Study the drawing (mm; zero at the part's minimum x, y, z) and answer. A direction names the side the tool comes from. Give positions to 0.01 mm unless a question says otherwise; leave off trailing zeros. Write each loop counter-clockwise with the first axis right and the second up, starting at its lowest first coordinate (ties: lowest second). Pieces come first, ordered by that corner, then holes. Notation, with made-up numbers: M -25,-27 L 10,-27 A12 ccw 10,-11 Z; hole C 36,-28.75 d4. An arc over 180 degrees is marked long. Use a Markdown table: item, result. Add a question column.
Item 1: Given P1, Ø2, axis at x = 5, z = 6.5, coming from the +Y side (3 decimals); P2, Ø4, axis at y = 2, z = 3.5, coming from the +X side; P3, Ø4, axis at y = 1, z = 6, coming from the -X side, each flat-ended and moving along its own axis, determine where each tip first touches the part or whether it passes through.
Item 2: A cutting plane is placed at A-A on z = 10.75. Determine the outline of the cut face in (x, y), then the cut area to 3 significant figures.
Item 3: Consider probe 1 along Y at (x, z) = (4, 3.5); probe 2 along Z at (x, y) = (6, 4.75); probe 3 along X at (y, z) = (4.5, 13). Determine where each line is inside the solid, lowest interval first. Write a range as [from, to].
Item 4: For the marked faces 1 and 2, determine the directions among +Z, -Z, +X, -X, +Y, -Y from which every point of the face is accessible in a straight line to the end or side of a thin tool.
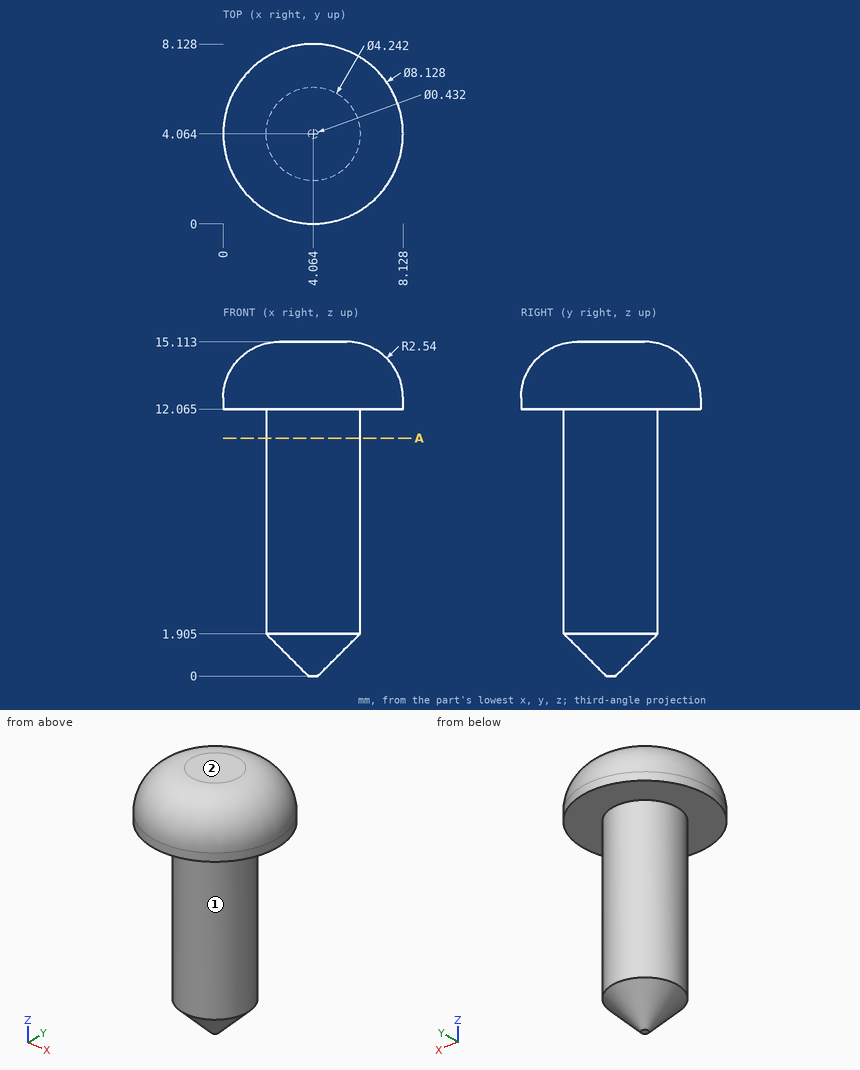
Filled in:
| question | item | result |
|---|---|---|
| 1 | P1 | y = 6.185 |
| 1 | P2 | x = 6.18 |
| 1 | P3 | x = 2.23 |
| 2 | outline | C 4.06,4.06 d4.24 |
| 2 | area | 14.1 mm² |
| 3 | probe 1 | [1.94, 6.18] |
| 3 | probe 2 | [1.84, 15.06] |
| 3 | probe 3 | [0.06, 8.07] |
| 4 | face 1 | -Z |
| 4 | face 2 | +Z, +X, -X, +Y, -Y |
